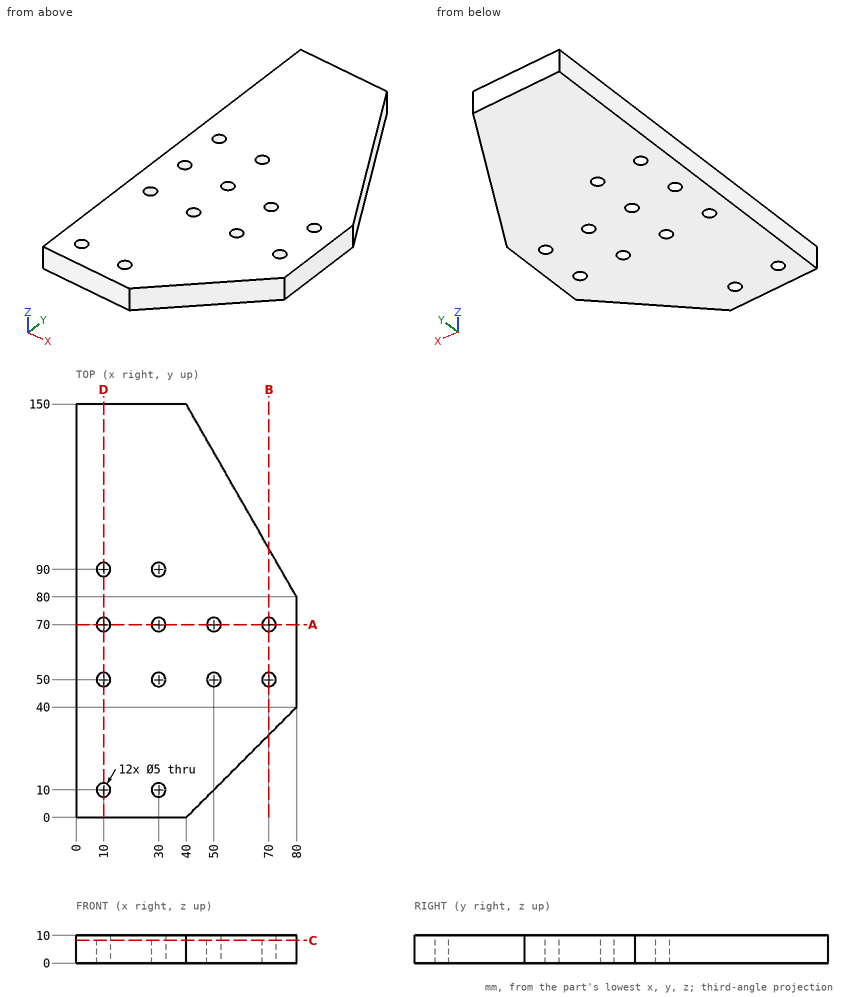
Job drawing, mm, ordinate dimensions from the low corner. One solid piece. Coordinates: 2 decimals unless noted, no trailing zeros. Order: outer loops, then holes, each group sorted by start corner. A loop starts at its lowest first (then second) coordinate and runs counter-clockwise, first axis right, second up. Notation, with made-up numbers: (45, -17) - (102, -17) arc R36 cw to (102, 21) - close; hole circle Ø6 at (10.5, -17). An arc over 180 degrees is marked (long way). Return JSON: item names as keys, results as strings. Group by question number.
1) Saw through at A-A, the plane y = 70. Write the cut outline in (x, z), plus the area to 3 significant figures.
2) Saw through at C-C, the plane z = 8.25. Count the separate pieces of the cut face and the enclosed holes in it, plus the area to 3 significant figures.
3) Probe line 1 (Y direction, x = 30, z = 7.75); line 2 (Y direction, x = 50, z = 7.5); line 3 (Y direction, x = 70, z = 6.25). List the from-to ranges inside material, lowest first. Write a range as from..to.
4) Saw through at D-D, the plane x = 10. Write the cut outline in (y, z).
5) Saw through at B-B, the plane x = 70. Write the cut outline in (y, z).
6) Flat gauge pins, fed straight in: P1, Ø3, axis at y = 119, z = 5.5, coming from the +X side; P2, Ø2, axis at y = 84, z = 2.5, coming from the +X side; P3, Ø6, axis at y = 85.5, z = 8.5, coming from the +X side. Where does each tip first touch, or does it go through?
Values found:
{
 "1": {"outline": "(0, 0) - (7.5, 0) - (7.5, 10) - (0, 10) - close; (12.5, 0) - (27.5, 0) - (27.5, 10) - (12.5, 10) - close; (32.5, 0) - (47.5, 0) - (47.5, 10) - (32.5, 10) - close; (52.5, 0) - (67.5, 0) - (67.5, 10) - (52.5, 10) - close; (72.5, 0) - (80, 0) - (80, 10) - (72.5, 10) - close", "area": "600 mm²"},
 "2": {"separate pieces": "1", "enclosed holes": "12", "area": "9,560 mm²"},
 "3": {"line 1": "y = 0..7.5, 12.5..47.5, 52.5..67.5, 72.5..87.5, 92.5..150", "line 2": "y = 10..47.5, 52.5..67.5, 72.5..132.5", "line 3": "y = 30..47.5, 52.5..67.5, 72.5..97.5"},
 "4": {"outline": "(0, 0) - (7.5, 0) - (7.5, 10) - (0, 10) - close; (12.5, 0) - (47.5, 0) - (47.5, 10) - (12.5, 10) - close; (52.5, 0) - (67.5, 0) - (67.5, 10) - (52.5, 10) - close; (72.5, 0) - (87.5, 0) - (87.5, 10) - (72.5, 10) - close; (92.5, 0) - (150, 0) - (150, 10) - (92.5, 10) - close"},
 "5": {"outline": "(30, 0) - (47.5, 0) - (47.5, 10) - (30, 10) - close; (52.5, 0) - (67.5, 0) - (67.5, 10) - (52.5, 10) - close; (72.5, 0) - (97.5, 0) - (97.5, 10) - (72.5, 10) - close"},
 "6": {"P1": "stops at x = 58.57", "P2": "stops at x = 78.29", "P3": "stops at x = 78.57"}
}
